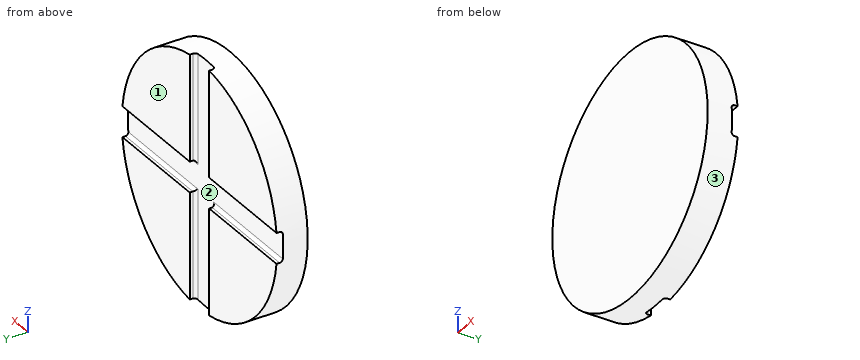
```python
from build123d import *

# Parameters (mm, degrees)
SKETCH1_R           = 40
BOSS_EXTRUDE1_DEPTH = 10
CUT_EXTRUDE2_DEPTH  = 2
FILLET1_R           = 1


with BuildPart() as part:
    # Sketch1 → Boss-Extrude1 (new body)
    with BuildSketch(Plane(origin=(0, 0, 0), x_dir=(1, 0, 0), z_dir=(0, 1, 0))):
        Circle(SKETCH1_R)
    extrude(amount=BOSS_EXTRUDE1_DEPTH)

    # Sketch7 → Cut-Extrude2 (cut)
    with BuildSketch(Plane(origin=(0, 10, 0), x_dir=(1, 0, 0), z_dir=(0, 1, 0))):
        with BuildLine():
            Line((-5, 39.686269666), (-5, 5))
            Line((-5, 5), (-39.686269666, 5))
            ThreePointArc((-39.686269666, 5), (-40, 0), (-39.686269666, -5))
            Line((-39.686269666, -5), (-5, -5))
            Line((-5, -5), (-5, -39.686269666))
            ThreePointArc((-5, -39.686269666), (0, -40), (5, -39.686269666))
            Line((5, -39.686269666), (5, -5))
            Line((5, -5), (39.686269666, -5))
            ThreePointArc((39.686269666, -5), (40, 0), (39.686269666, 5))
            Line((39.686269666, 5), (5, 5))
            Line((5, 5), (5, 39.686269666))
            ThreePointArc((5, 39.686269666), (0, 40), (-5, 39.686269666))
        make_face()
    extrude(amount=-CUT_EXTRUDE2_DEPTH, mode=Mode.SUBTRACT)

    # Fillet1
    fillet1_edges = [part.edges().sort_by_distance(p)[0] for p in [
        (5, 8, -22.343134833),
        (22.343134833, 8, -5),
        (22.343134833, 8, 5),
        (5, 8, 22.343134833),
        (-5, 8, 22.343134833),
        (-22.343134833, 8, 5),
        (-22.343134833, 8, -5),
        (-5, 8, -22.343134833),
    ]]
    fillet(fillet1_edges, radius=FILLET1_R)


solid = part.part
```
Check sheet for the modelled part. Datum: model origin and axes. Units: mm. Face numbers are marked on the shaded views. Round coordinates to 2 decimals unless told otherwise and drop trailing zeros. Order: outer loops, then holes, each group sorted by start corner. A loop starts at its lowest first (then second) coordinate and runs counter-clockwise, first axis right, second up.
1) Scan lines: line 1 (Y direction, x = -6.5, z = 0.5); line 2 (Z direction, x = 16.5, y = 8.25); line 3 (X direction, y = 9.5, z = 19). Record each from-to range of solid material in increasing order.
2) Section check D-D (x = 0). Record the boundary of the cut face in (y, z), and give its area (3 significant figures).
3) Section check B-B (x = -11.5). Record the boundary of the cut face in (y, z).
4) Section check A-A (z = 17). Record the boundary of the cut face in (x, y).
5) Mould release check, pull along Z, two halves, no side actions. Record for the marked faces 1, 2 and 3: +Z half, -Z half, draft (parallel to the pull), parting line (faces both ways), or undercut.
6) Section check C-C (y = 6.25). Record the boundary of the cut face in (x, z), and give its area (3 significant figures).
7) Go/stop test with flat-tipped pins: pin 1 Ø0.5 at (y, z) = (9.5, 14) entering from -X; pin 2 Ø0.8 at (y, z) = (9.5, -18.5) entering from +X; pin 3 Ø4 at (x, y) = (-14.5, 2) entering from -Z; pin 4 Ø1.5 at (x, z) = (-2, 4.5) entering from -Y. Record where each tip stops, or that it passes through.
Result:
1. line 1: y = 0 to 8
1. line 2: z = -36.44 to -4.66, 4.66 to 36.44
1. line 3: x = -35.2 to -5, 5 to 35.2
2. outline: (0, -40) - (8, -40) - (8, 40) - (0, 40) - close
2. area: 640 mm2
3. outline: (0, -38.31) - (10, -38.31) - (10, -5) - (9, -5) arc R1 cw to (8, -4) - (8, 4) arc R1 cw to (9, 5) - (10, 5) - (10, 38.31) - (0, 38.31) - close
4. outline: (-36.21, 0) - (36.21, 0) - (36.21, 10) - (5, 10) - (5, 9) arc R1 cw to (4, 8) - (-4, 8) arc R1 cw to (-5, 9) - (-5, 10) - (-36.21, 10) - close
5. face 1: draft
5. face 2: undercut
5. face 3: parting line
6. outline: circle Ø80 at (0, 0)
6. area: 5,030 mm2
7. pin 1: stops at x = -37.56
7. pin 2: stops at x = 35.67
7. pin 3: stops at z = -38
7. pin 4: stops at y = 0
